Geometry: final body of the model. Coordinates: model frame, mm. A direction names the side the tool comes from. Give positions to 0.01 mm unless a question says otherwise; leave off trailing zeros. Write each loop counter-clockwise with the first axis right and the second up, starting at its lowest first coordinate (ties: lowest second). Pieces come first, ordered by that corner, then holes.
from build123d import *

# Parameters (mm, degrees)
SKETCH1_W                = 75
SKETCH1_H                = 75
BOSS_EXTRUDE1_DEPTH      = 75
SKETCH2_R                = 5.35
CUT_EXTRUDE1_DEPTH       = 92.855865354
SKETCH5_R                = 8.5
CUT_EXTRUDE2_DEPTH       = 113.5
SKETCH7_R                = 20.71
SKETCH7_R_2              = 19.21
CUT_EXTRUDE3_DEPTH       = 3
SKETCH11_R               = 2
CUT_EXTRUDE4_DEPTH       = 10
SKETCH13_R               = 19.21
CUT_EXTRUDE7_DEPTH       = 50
SKETCH19_R               = 12.95
SKETCH19_R_2             = 11.9
CUT_EXTRUDE9_DEPTH       = 5
SKETCH20_R               = 2.25
CUT_EXTRUDE10_DEPTH      = 12.7
BOSS_EXTRUDE2_DEPTH      = 8
CUT_EXTRUDE14_DEPTH      = 99.496192858
CUT_EXTRUDE14_DEPTH_BACK = 99.496192858
SKETCH24_OUTSIDE_W       = 104.95
SKETCH24_OUTSIDE_H       = 104.95
SKETCH24_OUTSIDE_R       = 49.5


with BuildPart() as part:
    # Sketch1 → Boss-Extrude1 (new body)
    with BuildSketch(Plane(origin=(0, 0, 0), x_dir=(1, 0, 0), z_dir=(0, 1, 0))):
        Rectangle(SKETCH1_W, SKETCH1_H)
    extrude(amount=BOSS_EXTRUDE1_DEPTH)

    # Sketch2 → Cut-Extrude1 (cut, through all)
    with BuildSketch(Plane(origin=(0, 0, 0), x_dir=(-1, 0, 0), z_dir=(0, -1, 0))):
        with Locations(Location((0, 0, 0), (0, 0, 90))):
            Circle(SKETCH2_R)
    extrude(amount=-CUT_EXTRUDE1_DEPTH, mode=Mode.SUBTRACT)

    # Sketch5 → Cut-Extrude2 (cut, through all)
    with BuildSketch(Plane(origin=(37.5, 0, 0), x_dir=(0, 0, -1), z_dir=(1, 0, 0))):
        with Locations((0, 37.5)):
            Circle(SKETCH5_R)
    extrude(amount=-CUT_EXTRUDE2_DEPTH, mode=Mode.SUBTRACT)

    # Sketch7 → Cut-Extrude3 (cut)
    with BuildSketch(Plane.XZ):
        with Locations(Location((0, 0, 0), (0, 0, 270))):
            Circle(SKETCH7_R)
        with Locations(Location((0, 0, 0), (0, 0, 270))):
            Circle(SKETCH7_R_2, mode=Mode.SUBTRACT)
    cut_extrude3 = extrude(amount=-CUT_EXTRUDE3_DEPTH, mode=Mode.SUBTRACT)

    # Sketch11 → Cut-Extrude4 (cut)
    with BuildSketch(Plane.XZ):
        with Locations(Location((-33.75, 0, 0), (0, 0, 270))):
            Circle(SKETCH11_R)
        with Locations(Location((-23.864853865, 23.864853865, 0), (0, 0, 270))):
            Circle(SKETCH11_R)
        with Locations(Location((0, 33.75, 0), (0, 0, 270))):
            Circle(SKETCH11_R)
        with Locations(Location((23.864853865, 23.864853865, 0), (0, 0, 270))):
            Circle(SKETCH11_R)
        with Locations(Location((33.75, 0, 0), (0, 0, 270))):
            Circle(SKETCH11_R)
        with Locations(Location((23.864853865, -23.864853865, 0), (0, 0, 270))):
            Circle(SKETCH11_R)
        with Locations(Location((0, -33.75, 0), (0, 0, 270))):
            Circle(SKETCH11_R)
        with Locations(Location((-23.864853865, -23.864853865, 0), (0, 0, 270))):
            Circle(SKETCH11_R)
    cut_extrude4 = extrude(amount=-CUT_EXTRUDE4_DEPTH, mode=Mode.SUBTRACT)

    # Mirror1: Cut-Extrude3, Cut-Extrude4 across plane
    add(cut_extrude3.mirror(Plane.ZX.offset(37.5)), mode=Mode.SUBTRACT)
    add(cut_extrude4.mirror(Plane.ZX.offset(37.5)), mode=Mode.SUBTRACT)

    # Sketch13 → Cut-Extrude7 (cut)
    with BuildSketch(Plane(origin=(0, 75, 0), x_dir=(1, 0, 0), z_dir=(0, 1, 0))):
        with Locations(Location((0, 0, 0), (0, 0, 90))):
            Circle(SKETCH13_R)
    extrude(amount=-CUT_EXTRUDE7_DEPTH, mode=Mode.SUBTRACT)

    # Sketch19 → Cut-Extrude9 (cut)
    with BuildSketch(Plane(origin=(37.5, 0, 0), x_dir=(0, 0, -1), z_dir=(1, 0, 0))):
        with Locations((0, 37.5)):
            Circle(SKETCH19_R)
        with Locations((0, 37.5)):
            Circle(SKETCH19_R_2, mode=Mode.SUBTRACT)
    cut_extrude9 = extrude(amount=-CUT_EXTRUDE9_DEPTH, mode=Mode.SUBTRACT)

    # Sketch20 → Cut-Extrude10 (cut)
    with BuildSketch(Plane(origin=(37.5, 0, 0), x_dir=(0, 0, -1), z_dir=(1, 0, 0))):
        with Locations((-25, 37.5)):
            Circle(SKETCH20_R)
        with Locations((-12.5, 59.150635095)):
            Circle(SKETCH20_R)
        with Locations((12.5, 59.150635095)):
            Circle(SKETCH20_R)
        with Locations((25, 37.5)):
            Circle(SKETCH20_R)
        with Locations((12.5, 15.849364905)):
            Circle(SKETCH20_R)
        with Locations((-12.5, 15.849364905)):
            Circle(SKETCH20_R)
    cut_extrude10 = extrude(amount=-CUT_EXTRUDE10_DEPTH, mode=Mode.SUBTRACT)

    # Mirror4: Cut-Extrude9, Cut-Extrude10 across plane
    add(cut_extrude9.mirror(Plane.ZY), mode=Mode.SUBTRACT)
    add(cut_extrude10.mirror(Plane.ZY), mode=Mode.SUBTRACT)

    # Sketch25 → Boss-Extrude2 (add)
    with BuildSketch(Plane(origin=(0, 0, 0), x_dir=(1, 0, 0), z_dir=(0, 1, 0))):
        with BuildLine():
            Line((-37.5, 37.5), (-37.5, 2.740437921))
            ThreePointArc((-37.5, 2.740437921), (-26.587214973, 26.587214973), (-2.740437921, 37.5))
            Line((-2.740437921, 37.5), (-37.5, 37.5))
        make_face()
        with BuildLine():
            Line((37.5, 37.5), (2.740437921, 37.5))
            ThreePointArc((2.740437921, 37.5), (26.587214973, 26.587214973), (37.5, 2.740437921))
            Line((37.5, 2.740437921), (37.5, 37.5))
        make_face()
        with BuildLine():
            Line((-37.5, -37.5), (-2.740437921, -37.5))
            ThreePointArc((-2.740437921, -37.5), (-26.587214973, -26.587214973), (-37.5, -2.740437921))
            Line((-37.5, -2.740437921), (-37.5, -37.5))
        make_face()
        with BuildLine():
            Line((37.5, -37.5), (37.5, -2.740437921))
            ThreePointArc((37.5, -2.740437921), (26.587214973, -26.587214973), (2.740437921, -37.5))
            Line((2.740437921, -37.5), (37.5, -37.5))
        make_face()
    boss_extrude2 = extrude(amount=-BOSS_EXTRUDE2_DEPTH)

    # Mirror5: Boss-Extrude2 across plane
    add(boss_extrude2.mirror(Plane(origin=(0, 37.5, 0), x_dir=(0, 0, 1), z_dir=(0, -1, 0))))

    # Sketch24 outside → Cut-Extrude14 (cut, two sides: drawn at the far end of the back side and taken through both)
    with BuildSketch(Plane(origin=(0, 0, 0), x_dir=(1, 0, 0), z_dir=(0, 1, 0)).offset(-CUT_EXTRUDE14_DEPTH_BACK)):
        Rectangle(SKETCH24_OUTSIDE_W, SKETCH24_OUTSIDE_H)
        Circle(SKETCH24_OUTSIDE_R, mode=Mode.SUBTRACT)
    extrude(amount=CUT_EXTRUDE14_DEPTH + CUT_EXTRUDE14_DEPTH_BACK, mode=Mode.SUBTRACT)


solid = part.part
Q1. Pin query (flat end, axial travel): P1, Ø4.5, axis at x = 0, z = -33.75, coming from the -Y side; P2, Ø4.5, axis at x = 0, z = 33.75, coming from the +Y side; P3, Ø1.2, axis at x = -34, z = -0.5, coming from the +Y side. Return the tip coordinate at first contact, or that it passes through.
Filled sheet:
P1: stops at y = 0
P2: stops at y = 75
P3: stops at y = 65
Q2. Access query for faces 4 (the flat face through (-24.8, 59, -12)), 5 (the cylindrical face through (22.09, 70.07, 22.94)), 6 (the cylindrical face through (-26.85, -3.94, -26.32)). Directions: +Z, -Z, +X, -X, +Y, -Y. A direction counts if a zero-diameter tool reaches every point of the face in a straight line with its end or side. Return the directions, or none.
Filled sheet:
face 4: -X
face 5: +Y
face 6: -Y
Q3. Ray query, line 1 along Y through (x, z) = (-27.75, -12.5); line 2 along Y through (x, z) = (-16, -12.5); line 3 along Y through (x, z) = (21.5, -23.5). Return the intervals inside material, ascending.
Filled sheet:
line 1: y = 0 to 13.6, 18.1 to 56.9, 61.4 to 75
line 2: y = 3 to 72
line 3: y = 0 to 75
Q4. Section A-A on x = -33.75. Count the separate pieces of the cut face and the enclosed holes in it, plus the area to 3 significant figures.
Filled sheet:
separate pieces: 2
enclosed holes: 8
area: 5,580 mm2
Q5. Pull-direction query (Y, two-part tool) for faces 1 (the flat face through (4, 0, 4)), 2 (the cylindrical face through (-31.2, 14.5, -10.7)), 3 (the cylindrical face through (-5.223, 12.325, 1.16)); classes: released by +Y, released by -Y, zero draft, split by the parting line, or undercut.
Filled sheet:
face 1: released by -Y
face 2: undercut
face 3: zero draft
Q6. Section C-C on z = -33.75. Output: boundary loops of the cut face in (x, y), plus the area to 3 significant figures.
Filled sheet:
outline: (-36.21, -8) - (-16.57, -8) - (-16.57, 0) - (-2, 0) - (-2, 10) - (2, 10) - (2, 0) - (16.57, 0) - (16.57, -8) - (36.21, -8) - (36.21, 83) - (16.57, 83) - (16.57, 75) - (2, 75) - (2, 65) - (-2, 65) - (-2, 75) - (-16.57, 75) - (-16.57, 83) - (-36.21, 83) - close
area: 5,980 mm2
Q7. Section D-D on x = 15. Output: boundary loops of the cut face in (y, z), plus the area to 3 significant figures.
Filled sheet:
outline: (-8, -37.5) - (83, -37.5) - (83, -34.48) - (75, -34.48) - (75, -14.28) - (72, -14.28) - (72, -12) - (25, -12) - (25, 12) - (72, 12) - (72, 14.28) - (75, 14.28) - (75, 34.48) - (83, 34.48) - (83, 37.5) - (-8, 37.5) - (-8, 34.48) - (0, 34.48) - (0, 14.28) - (3, 14.28) - (3, 12) - (0, 12) - (0, -12) - (3, -12) - (3, -14.28) - (0, -14.28) - (0, -34.48) - (-8, -34.48) - close
area: 4,490 mm2
